Work out the finished part from the listing and answer in its coordinate system (mm). A direction names the side the tool comes from. Round coordinates to 2 decimals unless told otherwise and drop trailing zeros. Order: outer loops, then holes, each group sorted by start corner. A loop starts at its lowest first (then second) coordinate and runs counter-clockwise, first axis right, second up. Notation, with made-up numbers: (38.25, 51.25) -> (96.25, 51.25) arc R11 cw to (96.25, 67.25) -> close; hole circle Ø1 at (28, -33.75). An arc over 180 degrees is marked (long way). Use a Markdown table: item, result. Add a question column.
Item 1: A flat-ended cylindrical pin translates along its axis: P1, Ø1.5, axis at x = -53, z = -26, coming from the -Y side. Find the tip coordinate at first contact, or state that the pin passes through.
Item 2: Find the intervals of material crossed by L1, parallel to Z at x = 18, y = -33; L2, parallel to Z at x = 23.5, y = -29.5; L3, parallel to Z at x = 14, y = -33, in increasing order. Write a range as [from, to].
Item 3: A tool of negligible diameter and unlimited length cuts with its end or side. For faces 5 (the flat face through (1, 0, 1)), 6 (the flat face through (48, -35, 35)), from which of +Z, -Z, +X, -X, +Y, -Y can it reach the whole face along a straight path? Write none if from no direction.
Item 4: For a pull along Z with two mould halves and no side action, classify faces 1 (the flat face through (50, -32, -21)), 2 (the flat face through (-52, -19, 24)), 3 (the flat face through (-90, -20, 1)), 4 (the flat face through (1, -20, 60)) as +Z half, -Z half, draft (parallel to the pull), parting line (faces both ways), or undercut.
Item 5: A cutting plane is placed at B-B, the plane z = -48. Determine the outline of the cut face in (x, y).
Item 6: A cutting plane is placed at A-A, the plane y = -32.5. Give the number of separate pieces and of enclosed holes in the cut face, plus the area to 3 significant figures.
Item 7: A cutting plane is placed at D-D, the plane z = 8. Determine the outline of the cut face in (x, y).
Solid Edge part; units mm, degrees
sketch "Sketch1" plane through (0, 0, 0) normal (0, -1, 0) x (1, 0, 0)
  line L0 (90, -60) -> (90, 60)
  line L1 (90, 60) -> (-90, 60)
  line L2 (-90, 60) -> (-90, -60)
  line L3 (-90, -60) -> (90, -60)
extrude "Protrusion1" add sketch "Sketch1" along normal blind 40
sketch "Sketch2" plane through (0, -40, 0) normal (0, -1, 0) x (1, 0, 0)
  line L0 (-55, 50) -> (45, -50)
  line L1 (45, -50) -> (-55, -50)
  line L2 (-55, -50) -> (-55, 50)
  line L3 (-50, 37.9289) -> (-17.0711, 5)
  line L4 (-50, 5) -> (-17.0711, 5)
  line L5 (-50, 5) -> (-50, 37.9289)
  line L6 (-50, -15) -> (2.9289, -15)
  line L7 (2.9289, -15) -> (22.9289, -35)
  line L8 (5, -35) -> (22.9289, -35)
  line L9 (5, -41) -> (5, -35)
  line L10 (-2, -41) -> (5, -41)
  line L11 (-2, -35) -> (-2, -41)
  line L12 (-38, -35) -> (-2, -35)
  line L13 (-38, -41) -> (-38, -35)
  line L14 (-45, -41) -> (-38, -41)
  line L15 (-45, -35) -> (-45, -41)
  line L16 (-50, -35) -> (-45, -35)
  line L17 (-50, -35) -> (-50, -15)
  line L18 (55, -50) -> (-45, 50)
  line L19 (-45, 50) -> (55, 50)
  line L20 (55, 50) -> (55, -50)
  line L21 (-2.9289, 15) -> (-22.9289, 35)
  line L22 (-5, 35) -> (-22.9289, 35)
  line L23 (-5, 41) -> (-5, 35)
  line L24 (2, 41) -> (-5, 41)
  line L25 (2, 35) -> (2, 41)
  line L26 (38, 35) -> (2, 35)
  line L27 (38, 41) -> (38, 35)
  line L28 (45, 41) -> (38, 41)
  line L29 (45, 35) -> (45, 41)
  line L30 (50, 35) -> (45, 35)
  line L31 (50, 35) -> (50, 15)
  line L32 (50, 15) -> (-2.9289, 15)
  line L33 (50, -5) -> (17.0711, -5)
  line L34 (50, -37.9289) -> (17.0711, -5)
  line L35 (50, -5) -> (50, -37.9289)
extrude "VaciadoExtruido_1" cut sketch "Sketch2" against normal blind 11
sketch "Sketch3" plane through (-20, -29, 5) normal (0, -1, 0) x (1, 0, 0)
  line L0 (-35, 24) -> (-30, 24)
  line L1 (-30, 24) -> (-30, 14)
  line L2 (-30, 14) -> (-35, 14)
  line L3 (-35, 14) -> (-35, 24)
  line L4 (1.3604, 8.6396) -> (-2.1751, 5.1041)
  line L5 (-2.1751, 5.1041) -> (-9.2462, 12.1751)
  line L6 (-9.2462, 12.1751) -> (-5.7107, 15.7107)
  line L7 (-5.7107, 15.7107) -> (1.3604, 8.6396)
  line L8 (-35, -26) -> (-30, -26)
  line L9 (-30, -26) -> (-30, -36)
  line L10 (-30, -36) -> (-35, -36)
  line L11 (-35, -36) -> (-35, -26)
  line L12 (36.7157, -26.7157) -> (33.1802, -30.2513)
  line L13 (33.1802, -30.2513) -> (26.1091, -23.1802)
  line L14 (26.1091, -23.1802) -> (29.6447, -19.6447)
  line L15 (29.6447, -19.6447) -> (36.7157, -26.7157)
  line L16 (3.2843, 16.7157) -> (6.8198, 20.2513)
  line L17 (6.8198, 20.2513) -> (13.8909, 13.1802)
  line L18 (13.8909, 13.1802) -> (10.3553, 9.6447)
  line L19 (10.3553, 9.6447) -> (3.2843, 16.7157)
  line L20 (38.5843, -18.5843) -> (42.1198, -15.0488)
  line L21 (42.1198, -15.0488) -> (49.1909, -22.1198)
  line L22 (49.1909, -22.1198) -> (45.6554, -25.6554)
  line L23 (45.6554, -25.6554) -> (38.5843, -18.5843)
  line L24 (70, -24) -> (75, -24)
  line L25 (75, -24) -> (75, -34)
  line L26 (75, -34) -> (70, -34)
  line L27 (70, -34) -> (70, -24)
  line L28 (70, 26) -> (75, 26)
  line L29 (75, 26) -> (75, 16)
  line L30 (75, 16) -> (70, 16)
  line L31 (70, 16) -> (70, 26)
extrude "VaciadoExtruido_2" cut sketch "Sketch3" against normal blind 10
Reported:
| question | item | result |
|---|---|---|
| 1 | P1 | y = -19 |
| 2 | L1 | [-60, -50], [-35, -30.07], [-23, -13], [-5.93, -5], [15, 35], [50, 60] |
| 2 | L2 | [-60, -50], [-28.5, -18.5], [-11.43, -5], [15, 35], [50, 60] |
| 2 | L3 | [-60, -50], [-35, -26.07], [-19, -9], [15, 35], [50, 60] |
| 3 | face 5 | +Z, -Z, +X, -X, +Y |
| 3 | face 6 | -Y |
| 4 | face 1 | undercut |
| 4 | face 2 | undercut |
| 4 | face 3 | draft |
| 4 | face 4 | +Z half |
| 5 | outline | (-90, -40) -> (-55, -40) -> (-55, -29) -> (43, -29) -> (43, -40) -> (53, -40) -> (53, -29) -> (55, -29) -> (55, -40) -> (90, -40) -> (90, 0) -> (-90, 0) -> close |
| 6 | separate pieces | 5 |
| 6 | enclosed holes | 2 |
| 6 | area | 15,400 mm² |
| 7 | outline | (-90, -40) -> (-55, -40) -> (-55, -29) -> (-50, -29) -> (-50, -40) -> (-20.07, -40) -> (-20.07, -29) -> (-13, -29) -> (-13, -40) -> (-3, -40) -> (-3, -29) -> (55, -29) -> (55, -40) -> (90, -40) -> (90, 0) -> (-90, 0) -> close |
